The listing builds one solid part. Answer for the finished solid, in the listing's coordinates (mm). A direction names the side the tool comes from. Round coordinates to 2 decimals unless told otherwise and drop trailing zeros. Write each loop counter-clockwise with the first axis right and the second up, starting at its lowest first coordinate (ties: lowest second). Pieces come first, ordered by that corner, then holes.
(1) A cutting plane is placed at D-D, the plane z = 107.5. Give the vertices of the cut face in (x, y).
(2) Find the intervals of material crossed by probe 1 along X at (y, z) = (16, 0); probe 2 along Y at (x, z) = (1.75, 9.5); probe 3 along X at (y, z) = (33, 110), in increasing order.
(3) A cutting plane is placed at B-B, the plane x = 6.75. Give the vertices of the cut face in (y, z).
(4) Each of these flat-tipped pins is pushed along its axis until it touches: pin 1 Ø8 at (y, z) = (6, 100) entering from -X; pin 2 Ø10 at (y, z) = (34, 90) entering from +X; pin 3 Ø0.8 at (y, z) = (20.5, 116.5) entering from +X. Where does it stop, or does it pass through?
(5) For faces 1 (the face through (-8.876, 24.65, 32.818)), 2 (the face through (3.32, 25, 117)), 3 (the face through (12, 25, 109.773)), determine the directions among +Z, -Z, +X, -X, +Y, -Y from which every point of the face is accessible in a straight line to the end or side of a thin tool.
(6) A cutting plane is placed at A-A, the plane z = 0. Give the vertices of the cut face in (x, y).
(7) The mould has two halves that part along Y. Classify faces 4 (the face through (-0.54, 40.14, 2.44)), 5 (the face through (2, 20, 2)), 6 (the face through (-0.1, 50, 56)): +Y half, -Y half, draft (parallel to the pull), parting line (faces both ways), or undercut.
(8) A cutting plane is placed at C-C, the plane z = 77. Give the vertices of the cut face in (x, y).
from build123d import *

# Parameters (mm, degrees)
BOSS_EXTRUDE1_DEPTH     = 50
SKETCH2_R               = 2.5
CUT_EXTRUDE1_DEPTH      = 50
SKETCH3_W               = 40
SKETCH3_H               = 10
CUT_EXTRUDE2_DEPTH      = 10
CUT_EXTRUDE2_DEPTH_BACK = 50
SKETCH4_W               = 1.407970845
SKETCH4_H               = 1.5
CUT_EXTRUDE3_DEPTH      = 50
LPATTERN1_COUNT         = 20
LPATTERN1_PITCH         = 4.6


with BuildPart() as part:
    # Sketch1 → Boss-Extrude1 (new body)
    with BuildSketch(Plane(origin=(0, 0, 0), x_dir=(1, 0, 0), z_dir=(0, 1, 0))):
        with BuildLine():
            Line((9.367667652, -3.499543222), (0.000115688, -55.342775793))
            Line((0.000115688, -55.342775793), (10, -109.773324045))
            Line((10, -109.773324045), (14.389217383, -109.773324045))
            Line((14.389217383, -109.773324045), (14.389217383, -123.847521807))
            Line((14.389217383, -123.847521807), (10, -123.847521807))
            Line((10, -123.847521807), (3.320195055, -123.847521807))
            Line((3.320195055, -123.847521807), (3.320195055, -109.773324045))
            Line((3.320195055, -109.773324045), (-14.969009399, -55.342775793))
            Line((-14.969009399, -55.342775793), (-2.61095993, -9.653128417))
            ThreePointArc((-2.61095993, -9.653128417), (-4.56945593, 8.894946459), (9.367667652, -3.499543222))
        make_face()
    extrude(amount=BOSS_EXTRUDE1_DEPTH)

    # Sketch2 → Cut-Extrude1 (cut)
    with BuildSketch(Plane(origin=(0, 50, 0), x_dir=(1, 0, 0), z_dir=(0, 1, 0))):
        Circle(SKETCH2_R)
    extrude(amount=-CUT_EXTRUDE1_DEPTH, mode=Mode.SUBTRACT)

    # Sketch3 → Cut-Extrude2 (cut, two sides)
    with BuildSketch(Plane.XY) as cut_extrude2_sk:
        with Locations((10, 25)):
            Rectangle(SKETCH3_W, SKETCH3_H)
    extrude(amount=CUT_EXTRUDE2_DEPTH, mode=Mode.SUBTRACT)
    extrude(cut_extrude2_sk.sketch, amount=-CUT_EXTRUDE2_DEPTH_BACK, mode=Mode.SUBTRACT)

    # Sketch4 → Cut-Extrude3 (cut)
    with BuildSketch(Plane.XY.offset(123.847521807)):
        with Locations((13.685231961, 48.055062802)):
            Rectangle(SKETCH4_W, SKETCH4_H)
    cut_extrude3 = extrude(amount=-CUT_EXTRUDE3_DEPTH, mode=Mode.SUBTRACT)

    # LPattern1: Cut-Extrude3 ×20
    with Locations(*[(0, -i * LPATTERN1_PITCH, 0) for i in range(1, LPATTERN1_COUNT)]):
        add(cut_extrude3, mode=Mode.SUBTRACT)


solid = part.part
Solutions:
1. outline: (2.56, 0) - (9.58, 0) - (9.58, 50) - (2.56, 50) - close
2. probe 1: x = -10 to -2.5, 2.5 to 10
2. probe 2: y = 0 to 20, 30 to 50
2. probe 3: x = 3.32 to 14.39
3. outline: (0, -7.38) - (20, -7.38) - (20, 10) - (30, 10) - (30, -7.38) - (50, -7.38) - (50, 17.99) - (0, 17.99) - close; (0, 92.08) - (50, 92.08) - (50, 123.85) - (0, 123.85) - close
4. pin 1: stops at x = -1.31
4. pin 2: stops at x = 7.29
4. pin 3: stops at x = 12.98
5. face 1: -X, +Y, -Y
5. face 2: +Z, -X, +Y, -Y
5. face 3: -Z, +X, +Y, -Y
6. outline: (-10, 0) - (-2.5, 0) - (-2.5, 20) - (-10, 20) - close; (-10, 30) - (-2.5, 30) - (-2.5, 50) - (-10, 50) - close; (2.5, 0) - (10, 0) - (10, 20) - (2.5, 20) - close; (2.5, 30) - (10, 30) - (10, 50) - (2.5, 50) - close
7. face 4: draft
7. face 5: undercut
7. face 6: +Y half
8. outline: (-7.69, 0) - (3.98, 0) - (3.98, 50) - (-7.69, 50) - close
